Geometry: final body of the model. Coordinates: model frame, mm. Give positions to 0.01 mm unless a question says otherwise; leave off trailing zeros. Write each loop counter-clockwise with the first axis right and the second up, starting at its lowest first coordinate (ties: lowest second). Pieces come first, ordered by that corner, then holes. Notation, with made-up numbers: (28, 65) -> (51, 65) arc R27 cw to (51, 92) -> close; hole circle Ø7 at (88.25, -30.75). An arc over 180 degrees is marked (long way). Answer in a Markdown table with one row per item. Add a question column.
Item 1: Section query B-B on y = -7.5. Output: boundary loops of the cut face in (x, z), plus the area to 3 significant figures.
Item 2: Draft query along Y for faces 1 (the flat face through (23, -15, -3)), 2 (the cylindrical face through (22.78, -9.15, -3.03)), 3 (the flat face through (19.639, -6, -2)). Return one class per face: +Y half, -Y half, draft (parallel to the pull), parting line (faces both ways), or undercut.
Item 3: Section query A-A on z = -3.1. Output: boundary loops of the cut face in (x, y), plus the area to 3 significant figures.
Item 4: Section query C-C on x = 25.5. Output: boundary loops of the cut face in (y, z), plus the area to 3 significant figures.
Item 5: Material intervals for probe 1 along Z at (x, y) = (22.25, -7.5); probe 2 along Y at (x, z) = (21.75, -1.75); probe 3 along Y at (x, z) = (21.75, -3.5), sorted ascending. Write a range as from..to.
```python
from build123d import *

# Parameters (mm, degrees)
F0_W     = 6.2
F0_H     = 6.2
F1_DEPTH = 15
F2_R     = 1.65
F3_DEPTH = 6.2


# Not quite as in the source:
# - a feature names something its author has since deleted; it is built from what else it names


with BuildPart() as f1:
    # F0 (on Front) → F1 (new body)
    with BuildSketch(Plane.XZ):
        with Locations((22.738877362, -3.1)):
            Rectangle(F0_W, F0_H)
    extrude(amount=F1_DEPTH)

    # F2 (on face) → F3 (cut, through all)
    with BuildSketch(Plane.YZ.offset(25.838877362)):
        with Locations((-7.5, -3.1)):
            Circle(F2_R)
    extrude(amount=-F3_DEPTH, mode=Mode.SUBTRACT)


solid = f1.part
```
Findings below:
| question | item | result |
|---|---|---|
| 1 | outline | (19.64, -6.2) -> (25.84, -6.2) -> (25.84, -4.75) -> (19.64, -4.75) -> close; (19.64, -1.45) -> (25.84, -1.45) -> (25.84, 0) -> (19.64, 0) -> close |
| 1 | area | 18.0 mm^2 |
| 2 | face 1 | -Y half |
| 2 | face 2 | undercut |
| 2 | face 3 | draft |
| 3 | outline | (19.64, -15) -> (25.84, -15) -> (25.84, -9.15) -> (19.64, -9.15) -> close; (19.64, -5.85) -> (25.84, -5.85) -> (25.84, 0) -> (19.64, 0) -> close |
| 3 | area | 72.5 mm^2 |
| 4 | outline | (-15, -6.2) -> (0, -6.2) -> (0, 0) -> (-15, 0) -> close; hole circle Ø3.3 at (-7.5, -3.1) |
| 4 | area | 84.4 mm^2 |
| 5 | probe 1 | z = -6.2..-4.75, -1.45..0 |
| 5 | probe 2 | y = -15..-8.45, -6.55..0 |
| 5 | probe 3 | y = -15..-9.1, -5.9..0 |
